Here's how the part is built. I have some questions about the finished solid (model axes, mm). Coordinates: 2 decimals unless noted, no trailing zeros. Loops run counter-clockwise (first coordinate to the right, second up) from the corner with the lowest first, then second, coordinate; pieces in that order, holes last. Notation, with made-up numbers: M -1.5,-29.5 L 46.5,-29.5 A27 ccw 46.5,-13.5 Z; hole C -40,61 d7. An arc over 180 degrees is marked long. Use CSV: the item, a comma, the result in double quotes. Start each with the question number.
Q1. Please list where these lines run through material, in increasing order: probe 1 along Y at (x, z) = (0, -0.75); probe 2 along X at (y, z) = (-23, -0.6). Write a range as [from, to].
Q2. If we section it at A-A (y = 0): Please give me the cut outline in (x, z), and give its area (3 significant figures).
Q3. If we section it at C-C (z = -0.2): Please give me the cut outline in (x, y), and give its area (3 significant figures).
Q4. If we mould it in two halves opening along Y, with no side actions, what happens to faces 1 (the cylindrical face through (-3, 0.1, -0.5)), 2 (the flat face through (-6, 0, 0)), 3 (the cylindrical face through (24.859, 24.797, -0.493))? For each: +Y half, -Y half, draft (parallel to the pull), parting line (faces both ways), or undercut.
from build123d import *

# Parameters (mm, degrees)
PAD_DEPTH    = 1
SKETCH001_R  = 3
POCKET_DEPTH = 1.001


with BuildPart() as part:
    # Sketch → Pad (new body)
    with BuildSketch(Plane.XY):
        with BuildLine():
            Line((-26, 21.999982), (-26, -21.999982))
            ThreePointArc((-26, -21.999982), (-24.828421, -24.828421), (-21.999982, -26))
            Line((-21.999982, -26), (21.999982, -26))
            ThreePointArc((21.999982, -26), (24.828422, -24.828422), (26, -21.999982))
            Line((26, 21.999982), (26, -21.999982))
            ThreePointArc((26, 21.999982), (24.828422, 24.828422), (21.999982, 26))
            Line((-21.999982, 26), (21.999982, 26))
            ThreePointArc((-21.999982, 26), (-24.828427, 24.828427), (-26, 21.999982))
        make_face()
    extrude(amount=-PAD_DEPTH)

    # Sketch001 (on Face9 of Pad) → Pocket (cut, through all)
    with BuildSketch(Plane.XY):
        Circle(SKETCH001_R)
    extrude(amount=-POCKET_DEPTH, mode=Mode.SUBTRACT)


solid = part.part
Results below:
1,probe 1,"[-26, -3], [3, 26]"
1,probe 2,"[-25.87, 25.87]"
2,outline,"M -26,-1 L -3,-1 L -3,0 L -26,0 Z; M 3,-1 L 26,-1 L 26,0 L 3,0 Z"
2,area,"46.0 mm^2"
3,outline,"M -26,-22 A4 ccw -22,-26 L 22,-26 A4 ccw 26,-22 L 26,22 A4 ccw 22,26 L -22,26 A4 ccw -26,22 Z; hole C 0,0 d6"
3,area,"2,660 mm^2"
4,face 1,"undercut"
4,face 2,"draft"
4,face 3,"+Y half"
